Part print with two shaded views. Sizes in mm from the minimum x, y, z corner. Give positions to 0.01 mm unless a question says otherwise; leave off trailing zeros. Order: outer loops, then holes, each group sorted by start corner. A loop starts at its lowest first (then second) coordinate and runs counter-clockwise, first axis right, second up. Notation, with made-up numbers: (79, 5.5) -> (97, 5.5) arc R15 ccw to (97, 33.5) -> close; hole circle Ø6 at (69, 34.5). An arc over 180 degrees is marked (long way). Write item = value, one per line. Start each with the question number.
Item 1: Band-saw the part on A-A on x = 29.5. Count the separate pieces of the cut face and the enclosed holes in it, plus the area to 3 significant figures.
Item 2: Band-saw the part on D-D on z = 38.5. Write the cut outline in (x, y) (1 decimal).
Item 3: Band-saw the part on C-C on x = 43.5. Write the cut outline in (y, z) (1 decimal).
Item 4: Drill centre lines: line 1 along Z through (x, y) = (28, 2.8) (1 decimal); line 2 along Z through (x, y) = (43.5, 2.95) (1 decimal); line 3 along X through (y, z) = (0.45, 27) (1 decimal). Where is each one in solid material? Low to high.
Item 5: Flat gauge pins, fed straight in: P1, Ø1.5, axis at y = 2.5, z = 30.5, coming from the +X side; P2, Ø1, axis at x = 8.5, y = 1.5, coming from the -Z side; P3, Ø1, axis at x = 24, y = 1, coming from the +Z side. Where does each tip first touch, or does it go through?
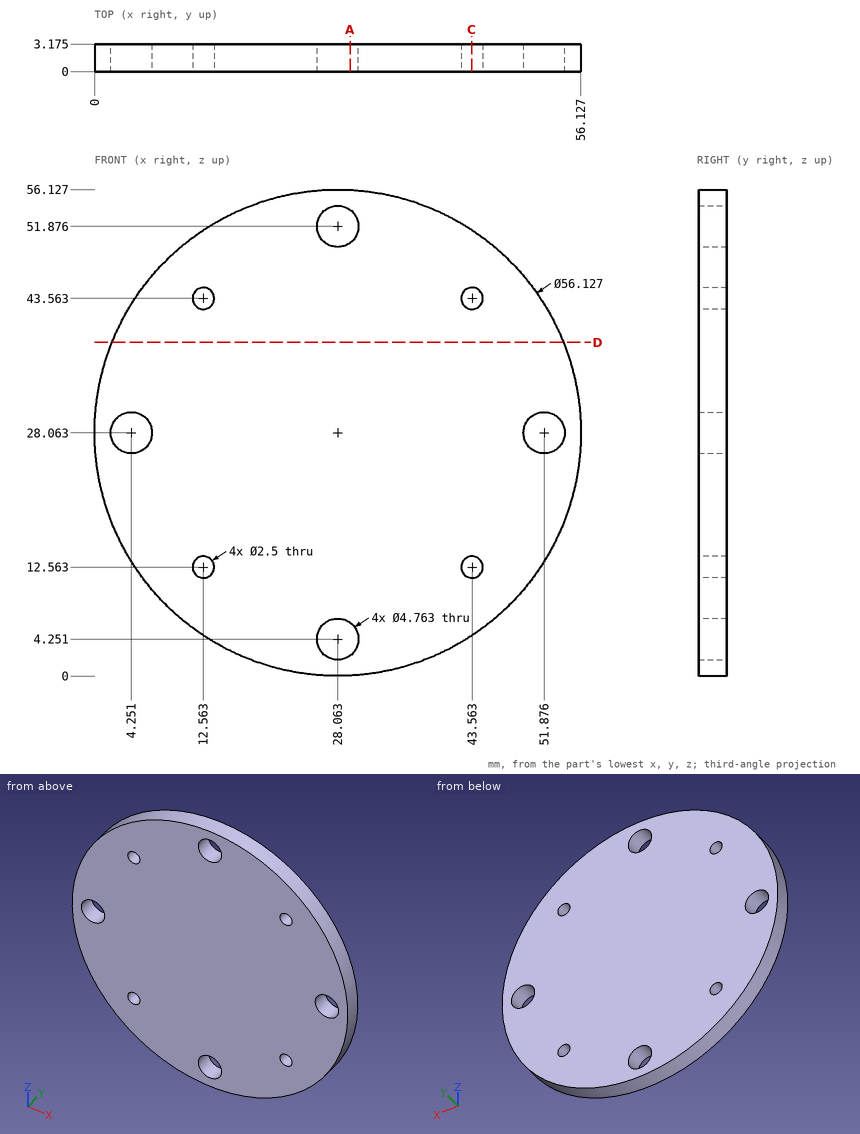
Values found:
q1.separate_pieces = 3
q1.enclosed_holes = 0
q1.area = 154 mm^2
q2.outline = (2, 0) -> (54.1, 0) -> (54.1, 3.2) -> (2, 3.2) -> close
q3.outline = (0, 4.6) -> (3.2, 4.6) -> (3.2, 11.3) -> (0, 11.3) -> close; (0, 13.8) -> (3.2, 13.8) -> (3.2, 42.3) -> (0, 42.3) -> close; (0, 44.8) -> (3.2, 44.8) -> (3.2, 51.5) -> (0, 51.5) -> close
q4.line_1 = 0 to 1.9, 6.6 to 49.5, 54.3 to 56.1
q4.line_2 = 4.6 to 11.3, 13.8 to 42.3, 44.8 to 51.5
q4.line_3 = 0 to 2.1, 6.4 to 49.7, 54 to 56.1
q5.P1 = 56.08
q5.P2 = 7.47
q5.P3 = 55.9
